from build123d import *

# Parameters (mm, degrees)
BOSS_EXTRUDE1_DEPTH = 2.5
SKETCH3_R           = 10
BOSS_EXTRUDE2_DEPTH = 11
SKETCH4_R           = 6
BOSS_EXTRUDE3_DEPTH = 6
M8_TAPPED_HOLE1_D   = 6.8
SKETCH7_W           = 10
SKETCH7_H           = 10
CUT_EXTRUDE1_DEPTH  = 67.970142601


with BuildPart() as part:
    # Sketch2 → Boss-Extrude1 (new, symmetric)
    with BuildSketch(Plane.XY):
        with BuildLine():
            Line((-9.539392014, -3), (-2.384848004, -25.75))
            ThreePointArc((-2.384848004, -25.75), (0, -27.5), (2.384848004, -25.75))
            Line((2.384848004, -25.75), (9.539392014, -3))
            ThreePointArc((9.539392014, -3), (9.92690409, -1.206886566), (9.980334012, 0.626843686))
            Line((9.980334012, 0.626843686), (6, 64))
            Line((6, 64), (-6, 64))
            Line((-6, 64), (-9.980334012, 0.626843686))
            ThreePointArc((-9.980334012, 0.626843686), (-9.92690409, -1.206886566), (-9.539392014, -3))
        make_face()
    extrude(amount=BOSS_EXTRUDE1_DEPTH, both=True)

    # Sketch3 → Boss-Extrude2 (add)
    with BuildSketch(Plane.XY.offset(2.5)):
        with Locations(Location((0, 0, 0), (0, 0, 176.406094003))):
            Circle(SKETCH3_R)
    extrude(amount=-BOSS_EXTRUDE2_DEPTH)

    # Sketch4 → Boss-Extrude3 (add)
    with BuildSketch(Plane.XY.offset(2.5)):
        with Locations((0, 50)):
            Circle(SKETCH4_R)
    extrude(amount=BOSS_EXTRUDE3_DEPTH)

    # M8 Tapped Hole1 (through all)
    with Locations(Plane.XY.offset(8.5)):
        with Locations((0, 50)):
            Hole(M8_TAPPED_HOLE1_D / 2)

    # Sketch7 → Cut-Extrude1 (cut, through all)
    with BuildSketch(Plane(origin=(0, 0, -8.5), x_dir=(-1, 0, 0), z_dir=(0, 0, -1))):
        Rectangle(SKETCH7_W, SKETCH7_H)
    extrude(amount=-CUT_EXTRUDE1_DEPTH, mode=Mode.SUBTRACT)

    # Sketch8 → Revolve1 (revolve)
    with BuildSketch(Plane.XY, mode=Mode.PRIVATE) as revolve1_sk:
        with BuildLine():
            Line((0, 64), (-7, 64))
            Line((-7, 64), (-7, 67))
            Line((-7, 67), (-4.5, 67))
            Line((-4.5, 67), (-8, 99))
            ThreePointArc((-8, 99), (-4.472135955, 101.94427191), (0, 103))
            Line((0, 103), (0, 64))
        make_face()
    revolve(revolve1_sk.sketch.rotate(Axis((0, 0, 0), (0, 1, 0)), 270), axis=Axis((0, 0, 0), (0, 1, 0)))


solid = part.part
Geometry check sheet. Reference: the model listing, model coordinates, mm. A direction names the side the tool comes from. Coordinates: 2 decimals unless noted, no trailing zeros. Order: outer loops, then holes, each group sorted by start corner. A loop starts at its lowest first (then second) coordinate and runs counter-clockwise, first axis right, second up. Notation, with made-up numbers: (-27, 2) -> (-11, 2) arc R32 cw to (-11, 41) -> close; hole circle Ø10 at (35, 50.25). An arc over 180 degrees is marked (long way). Use a Markdown table: item, result. Add a question column.
1. Cross-section at A-A (z = 0). Enter the section's corners in (x, y), and give its area (3 significant figures).
2. Cross-section at B-B (x = 0). Enter the section's corners in (y, z).
3. Cross-section at C-C (y = 50). Enter the section's corners in (x, z), and give its area (3 significant figures).
4. Mould release check, pull along X, two halves, no side actions. Record for faces 5 (the face through (0, -5, -3)), 6 (the face through (0, 33, -2.5)), 7 (the face through (6.834, 65.521, 1.517)): pulls with the +X half, pulls with the -X half, needs draft (parallel to the pull), parting line crosses it, or undercut.
5. Material ranges on L1, parallel to Y at x = 0, z = 0; L2, parallel to Y at x = 0, z = 1.5; L3, parallel to Z at x = 0.75, y = 6.5, recorded low to high.
6. Set-up check for faces 1 (the face through (0, 5, -3)), 2 (the face through (-7.962, 32.757, 0.035)), 3 (the face through (5, 67, 0)), 4 (the face through (0.678, -9.977, -4.145)): record each of +Z, -Z, +X, -X, +Y, -Y from which the full face is reachable in a straight line by a thin tool's end or side.
7. Cross-section at D-D (y = 90.5). Enter the section's corners in (x, z).
8. Go/stop test with flat-tipped pins: pin 1 Ø1.5 at (y, z) = (61.5, 5) entering from -X; pin 2 Ø5 at (y, z) = (2, -2.5) entering from -X; pin 3 Ø4 at (x, z) = (1.5, -2) entering from +Y; pin 4 Ø8 at (x, y) = (0, 50) entering from -Z. Record where each tip stops, or that it passes through.
Filled sheet:
| question | item | result |
|---|---|---|
| 1 | outline | (-9.98, 0.63) arc R10 ccw to (-9.54, -3) -> (-2.38, -25.75) arc R2.5 ccw to (2.38, -25.75) -> (9.54, -3) arc R10 ccw to (9.98, 0.63) -> (6, 64) -> (7, 64) -> (7, 67) -> (4.5, 67) -> (8, 99) arc R10 ccw to (-8, 99) -> (-4.5, 67) -> (-7, 67) -> (-7, 64) -> (-6, 64) -> close; hole (-5, -5) -> (5, -5) -> (5, 5) -> (-5, 5) -> close; hole circle Ø6.8 at (0, 50) |
| 1 | area | 1,710 mm2 |
| 2 | outline | (-27.5, -2.5) -> (-10, -2.5) -> (-10, -8.5) -> (-5, -8.5) -> (-5, 2.5) -> (-27.5, 2.5) -> close; (5, -8.5) -> (10, -8.5) -> (10, -2.5) -> (46.6, -2.5) -> (46.6, 8.5) -> (44, 8.5) -> (44, 2.5) -> (5, 2.5) -> close; (53.4, -2.5) -> (64, -2.5) -> (64, -7) -> (67, -7) -> (67, -4.5) -> (99, -8) arc R10 ccw to (99, 8) -> (67, 4.5) -> (67, 7) -> (64, 7) -> (64, 2.5) -> (56, 2.5) -> (56, 8.5) -> (53.4, 8.5) -> close |
| 3 | outline | (-6.88, -2.5) -> (-3.4, -2.5) -> (-3.4, 8.5) -> (-6, 8.5) -> (-6, 2.5) -> (-6.88, 2.5) -> close; (3.4, -2.5) -> (6.88, -2.5) -> (6.88, 2.5) -> (6, 2.5) -> (6, 8.5) -> (3.4, 8.5) -> close |
| 3 | area | 66.0 mm2 |
| 4 | face 5 | undercut |
| 4 | face 6 | needs draft |
| 4 | face 7 | parting line crosses it |
| 5 | L1 | -27.5 to -5, 5 to 46.6, 53.4 to 103 |
| 5 | L2 | -27.5 to -5, 5 to 46.6, 53.4 to 102.89 |
| 5 | L3 | -8.5 to 2.5 |
| 6 | face 1 | +Z, -Z |
| 6 | face 2 | +Z, -Z, -X |
| 6 | face 3 | none |
| 6 | face 4 | -Z |
| 7 | outline | circle Ø14.14 at (0, 0) |
| 8 | pin 1 | through |
| 8 | pin 2 | x = -10 |
| 8 | pin 3 | y = 102.99 |
| 8 | pin 4 | z = -2.5 |
